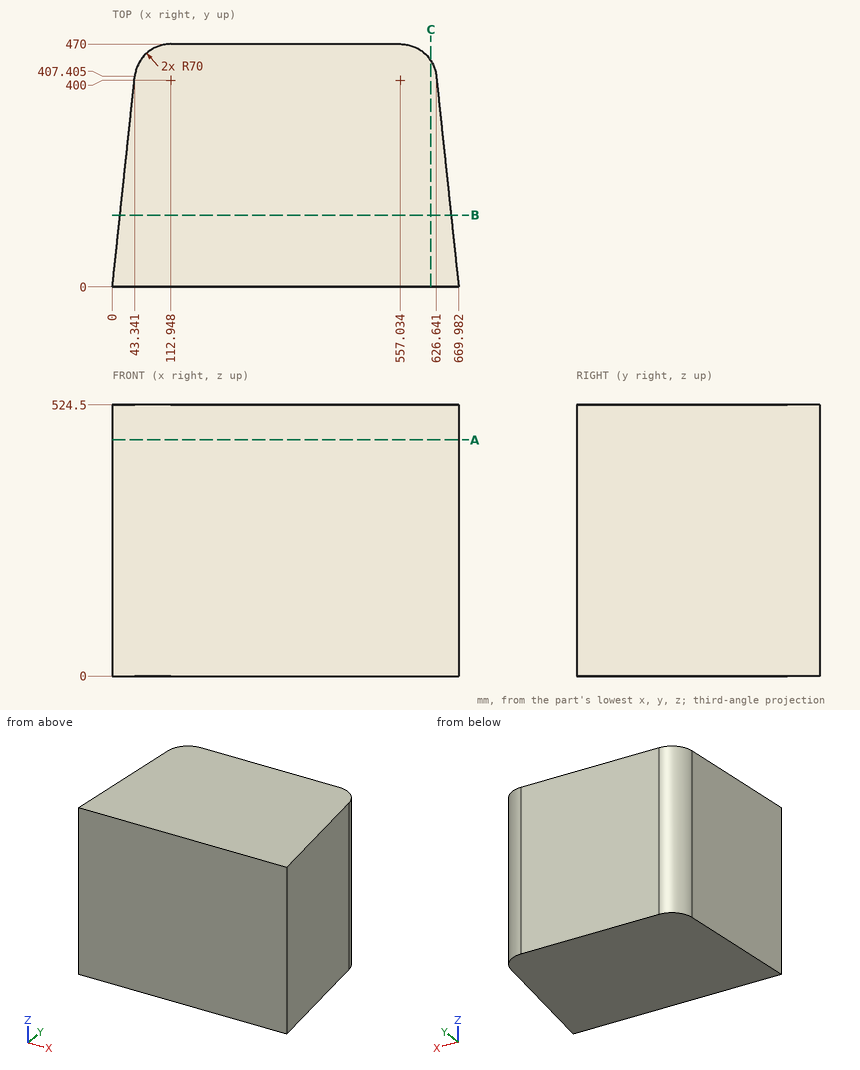
Verification items for this drawing (mm, ordinates from the low corner). Coordinates: 2 decimals unless noted, no trailing zeros. Order: outer loops, then holes, each group sorted by start corner. A loop starts at its lowest first (then second) coordinate and runs counter-clockwise, first axis right, second up. Notation, with made-up numbers: M 73,-4 L 128,-4 A31 ccw 128,27 Z; hole C 77,16 d5. An arc over 180 degrees is marked long. Use CSV: the item, a comma, the result in double quotes.
Item 1: Cross-section at B-B on y = 139. Record the cut outline in (x, z) (1 decimal), then the cut area to 3 significant figures.
Returned:
outline,"M 14.8,0 L 655.2,0 L 655.2,524.5 L 14.8,524.5 Z"
area,"336,000 mm2"
Item 2: Cross-section at A-A on z = 457. Record the cut outline in (x, y) (1 decimal).
Returned:
outline,"M 0,0 L 670,0 L 626.6,407.4 A70 ccw 557,470 L 112.9,470 A70 ccw 43.3,407.4 Z"
Item 3: Cross-section at C-C on x = 616. Record the cut outline in (y, z), then the cut area to 3 significant figures.
Returned:
outline,"M 0,0 L 437.72,0 L 437.72,524.5 L 0,524.5 Z"
area,"230,000 mm2"
Item 4: Gauge pin test, flat ends, axial feed: pin 1 Ø3 at (y, z) = (252, 241) entering from -X; pin 2 Ø1 at (y, z) = (216.5, 392) entering from -X; pin 3 Ø12 at (y, z) = (284, 283) entering from +X. Record the tip position at first contact, or that the pin passes through.
Returned:
pin 1,"stops at x = 26.65"
pin 2,"stops at x = 22.98"
pin 3,"stops at x = 640.41"
Item 5: Thickness scan on line 1 along X through (y, z) = (248, 424); line 2 along X through (y, z) = (57.5, 245) (1 decimal); line 3 along Y through (x, z) = (101.5, 429). Record the ranges inside material, lowest first.
Returned:
line 1,"x = 26.38 to 643.6"
line 2,"x = 6.1 to 663.9"
line 3,"y = 0 to 469.06"
